Check sheet for the drawn part. Datum: minimum x, y, z corner. Units: mm. A direction names the side the tool comes from. Round coordinates to 2 decimals unless told otherwise and drop trailing zeros. Write each loop counter-clockwise with the first axis right and the second up, starting at its lowest first coordinate (ties: lowest second). Pieces come first, ordered by that corner, then holes.
Item 1: Cross-section at D-D on x = 3. Enter the section's corners in (y, z).
Item 2: Cross-section at C-C on z = 2.75. Enter the section's corners in (x, y), plus the area to 3 significant figures.
Item 3: Release check for a two-part mould opening along X. For the marked faces 1, 2 and 3 record: +X half, -X half, draft (parallel to the pull), parting line (faces both ways), or undercut.
Item 4: Cross-section at A-A on x = 11. Enter the section's corners in (y, z).
Item 5: Tool access check on the marked faces 4, 5 and 6. Record the directions out of +Z, -Z, +X, -X, +Y, -Y that give a thin tool (end or side, any length) a straight path to the whole face; none if there is none.
Item 6: Cross-section at B-B on y = 20. Enter the section's corners in (x, z), plus the area to 3 significant figures.
Item 7: Go/stop test with flat-tipped pins: pin 1 Ø5 at (x, y) = (11, 11) entering from +Z; pin 2 Ø4 at (x, z) = (5.5, 11.5) entering from +Y; pin 3 Ø6 at (x, z) = (11, 12.5) entering from -Y; pin 4 Ø4.5 at (x, y) = (19, 11) entering from +Z. Record where each tip stops, or that it passes through.
Item 8: Material ranges on line 1 (Y direction, x = 11, z = 4.1); line 2 (Z direction, x = 3.5, y = 6); line 3 (Y direction, x = 11, z = 8), recorded low to high.
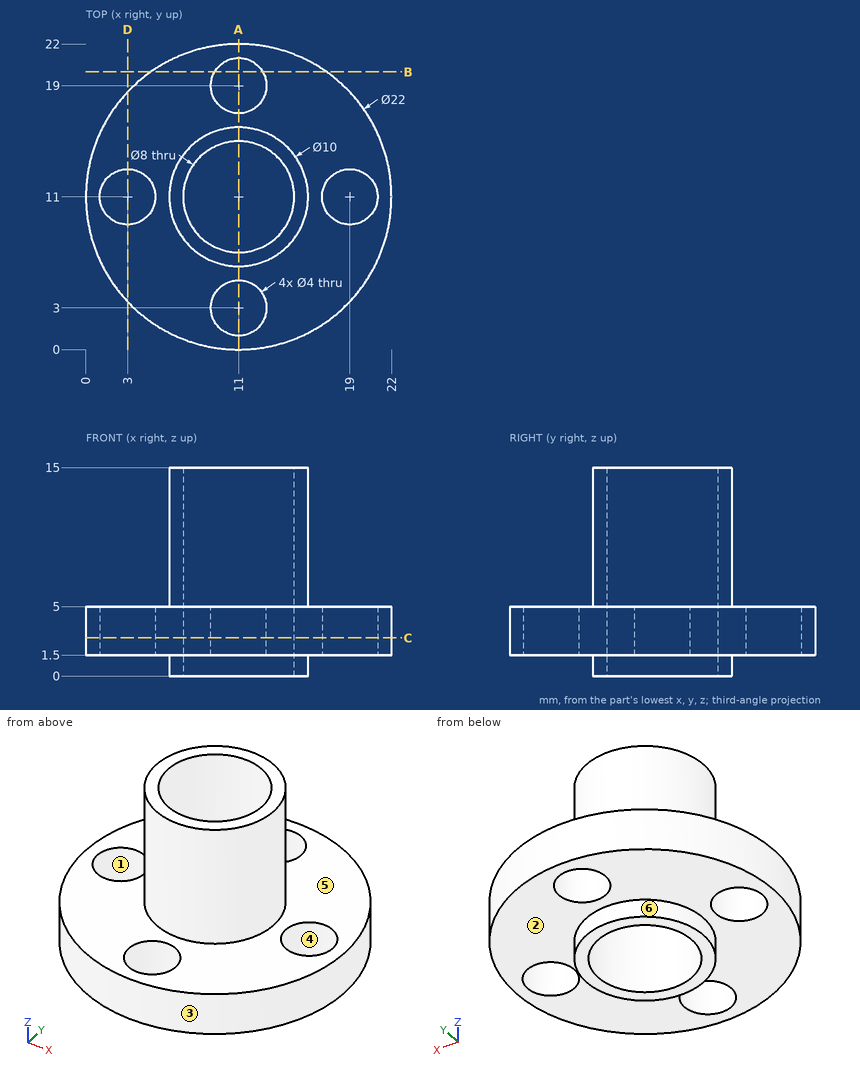
Response values:
1. outline: (3.45, 1.5) - (9, 1.5) - (9, 5) - (3.45, 5) - close; (13, 1.5) - (18.55, 1.5) - (18.55, 5) - (13, 5) - close
2. outline: circle Ø22 at (11, 11); hole circle Ø4 at (3, 11); hole circle Ø8 at (11, 11); hole circle Ø4 at (11, 3); hole circle Ø4 at (11, 19); hole circle Ø4 at (19, 11)
2. area: 280 mm2
3. face 1: undercut
3. face 2: draft
3. face 3: parting line
4. outline: (0, 1.5) - (1, 1.5) - (1, 5) - (0, 5) - close; (5, 1.5) - (6, 1.5) - (6, 0) - (7, 0) - (7, 15) - (6, 15) - (6, 5) - (5, 5) - close; (15, 0) - (16, 0) - (16, 1.5) - (17, 1.5) - (17, 5) - (16, 5) - (16, 15) - (15, 15) - close; (21, 1.5) - (22, 1.5) - (22, 5) - (21, 5) - close
5. face 4: +Z, -Z
5. face 5: +Z
5. face 6: -Z
6. outline: (4.68, 1.5) - (9.27, 1.5) - (9.27, 5) - (4.68, 5) - close; (12.73, 1.5) - (17.32, 1.5) - (17.32, 5) - (12.73, 5) - close
6. area: 32.1 mm2
7. pin 1: passes through
7. pin 2: stops at y = 14.57
7. pin 3: stops at y = 6
7. pin 4: stops at z = 5
8. line 1: y = 0 to 1, 5 to 7, 15 to 17, 21 to 22
8. line 2: z = 1.5 to 5
8. line 3: y = 6 to 7, 15 to 16
